Geometry: final body of the model. Coordinates: model frame, mm. A direction names the side the tool comes from. Give positions to 0.01 mm unless a question says otherwise; leave off trailing zeros. Order: outer loops, then holes, each group sorted by start corner. A loop starts at its lowest first (then second) coordinate and runs counter-clockwise, first axis right, second up. Notation, with made-up numbers: M 61,30 L 85,30 A11 ccw 85,47 Z; hole C 66,-24 d5. An arc over 180 degrees is marked long. Use CSV: the item, a comma, the result in double quotes.
```python
from build123d import *

# Parameters (mm, degrees)
F1_DEPTH   = 60
F2_C1_SIZE = 9.9999


# Not quite as in the source:
# - a fillet or chamfer is up to 0.001 mm smaller than in the source, because OpenCascade refuses the exact size


with BuildPart() as f1:
    # F0 (on Right) → F1 (new body)
    with BuildSketch(Plane.YZ):
        Polygon((-4, 5), (-5, 5), (-5, -5), (5, -5), (5, 5), (4, 5), (4, -4), (-4, -4), align=None)
    extrude(amount=F1_DEPTH)

    # F2: chamfer of 10 on 2 edges, made by hand

    # F2_c1 (size 10 in the source; OpenCascade refuses exactly that, so slightly less here)
    f2_c1_edges = [f1.edges().sort_by_distance(p)[0] for p in [
        (60, -4.5, 5),
    ]]
    chamfer(f2_c1_edges, length=F2_C1_SIZE)


solid = f1.part
```
1. Section D-D, the plane z = 1.5. Return the cut outline in (x, y).
Answer:
outline,"M 0,-5 L 53.5,-5 L 53.5,-4 L 0,-4 Z; M 0,4 L 53.5,4 L 53.5,5 L 0,5 Z"
2. Section A-A, the plane z = 4. Return the cut outline in (x, y), plus the area to 3 significant figures.
Answer:
outline,"M 0,-5 L 51,-5 L 51,-4 L 0,-4 Z; M 0,4 L 51,4 L 51,5 L 0,5 Z"
area,"102 mm2"
3. Line query: line 1 (Y direction, x = 39.5, z = 3); line 2 (Z direction, x = 41.5, y = -0.5); line 3 (X direction, y = -4.5, z = 3.25). Output: solid intervals per line, ascending.
Answer:
line 1,"-5 to -4, 4 to 5"
line 2,"-5 to -4"
line 3,"0 to 51.75"
4. Pin query (flat end, axial travel): pin 1 Ø1 at (y, z) = (0, -2.5) entering from +X; pin 2 Ø4 at (x, y) = (29.5, 1.5) entering from +Z. Return the tip coordinate at first contact, or that it passes through.
Answer:
pin 1,"through"
pin 2,"z = -4"
5. Section B-B, the plane x = 13. Return the cut outline in (y, z).
Answer:
outline,"M -5,-5 L 5,-5 L 5,5 L 4,5 L 4,-4 L -4,-4 L -4,5 L -5,5 Z"
6. Pull-direction query (Y, two-part tool) for faces 3 (the face through (29, 0, -4)), 4 (the face through (30, 0, -5)), 5 (the face through (30, -5, 0)), 6 (the face through (30, 5, 0)); classes: +Y half, -Y half, draft (parallel to the pull), parting line (faces both ways), or undercut.
Answer:
face 3,"undercut"
face 4,"draft"
face 5,"-Y half"
face 6,"+Y half"
7. Reachability of faces 1 (the face through (24.7, -4.5, 5)), 2 (the face through (29, -4, 0)) from +Z, -Z, +X, -X, +Y, -Y: full face, straight path, thin tool, end or side. Return the list, or none.
Answer:
face 1,"+Z, +X, -X, +Y, -Y"
face 2,"+Z, +X, -X"
